Autodesk Inventor part; units mm, degrees
ref_plane "YZ Plane" through (0, 0, 0) normal (1, 0, 0) x (0, 1, 0)
ref_plane "XZ Plane" through (0, 0, 0) normal (0, 1, 0) x (-1, 0, 0)
ref_plane "XY Plane" through (0, 0, 0) normal (0, 0, 1) x (1, 0, 0)
sketch "Sketch1" plane through (0, 0, 0) normal (0, 0, 1) x (1, 0, 0)
  circle A0 centre (190.0545, 3.9636) radius 5.5
  circle A1 centre (-96.9878, 447.3295) radius 5.5
  arc A2 (177.463, -4.1883) -> (202.646, 12.1156) centre (190.0545, 3.9636) ccw
  arc A3 (-84.3963, 455.4815) -> (-109.5793, 439.1776) centre (-96.9878, 447.3295) ccw
  line L0 (-84.3963, 455.4815) -> (202.646, 12.1156)
  line L1 (177.463, -4.1883) -> (-109.5793, 439.1776)
  circle A4 centre (190.0545, 3.9636) radius 5.5
  circle A5 centre (-96.9878, 447.3295) radius 5.5
  point P0 (0, 0)
  dimension "d2" = 30
  dimension "d3" = 30
  dimension "d4" = 11
  dimension "d5" = 11
extrude "Extrusion2" add sketch "Sketch1" along normal blind 6
properties material "Steel, Mild"
Input: part model. Units: mm. Frame: model coordinates. Give positions to 0.01 mm unless a question says otherwise; leave off trailing zeros. Loops run counter-clockwise (first coordinate to the right, second up) from the corner with the lowest first, then second, coordinate; pieces in that order, holes last. Notation, with made-up numbers: M 76,77 L 84,77 A20 ccw 84,102 Z; hole C 89.25,77.25 d4. An arc over 180 degrees is marked long. Use CSV: the item, a comma, the result in double quotes.
(1) Pin query (flat end, axial travel): P1, Ø2, axis at x = 9.5, z = 5.5, coming from the -Y side; P2, Ø1.5, axis at x = 135.5, z = 2, coming from the +Y side; P3, Ø1.5, axis at x = 47, z = 1.5, coming from the -Y side. Return the tip coordinate at first contact, or that it passes through.
Outcome:
P1,"stops at y = 253.7"
P2,"stops at y = 116.99"
P3,"stops at y = 196.17"
(2) Pull-direction query (X, two-part tool) for faces 1 (the face through (57.116, 236.902, 2.958)), 2 (the face through (46, 227, 0)), 3 (the face through (195.3, 2.31, 2.96)); classes: pulls with the +X half, pulls with the -X half, needs draft (parallel to the pull), parting line crosses it, or undercut.
Outcome:
face 1,"pulls with the +X half"
face 2,"needs draft"
face 3,"undercut"
(3) Material intervals for L1, parallel to Y at x = 23, z = 2.55; L2, parallel to Y at x = -64, z = 1.3; L3, parallel to X at y = 316, z = 3.6, sorted ascending. Write a range as [from, to].
Outcome:
L1,"y = [234.4, 289.6]"
L2,"y = [368.78, 423.98]"
L3,"x = [-29.83, 5.91]"
(4) Section C-C, the plane x = 48. Return loops of the section in (y, z), plus the area to 3 significant figures.
Outcome:
outline,"M 195.78,0 L 250.98,0 L 250.98,6 L 195.78,6 Z"
area,"331 mm²"
(5) Section A-A, the plane z = 3.75. Return loops of the section in (x, y), plus the area to 3 significant figures.
Outcome:
outline,"M -109.58,439.18 L 177.46,-4.19 A15 ccw 202.65,12.12 L -84.4,455.48 A15 ccw Z; hole C -96.99,447.33 d11; hole C 190.05,3.96 d11"
area,"16,400 mm²"
(6) Section B-B, the plane y = 31. Return loops of the section in (x, z), plus the area to 3 significant figures.
Outcome:
outline,"M 154.68,0 L 190.42,0 L 190.42,6 L 154.68,6 Z"
area,"214 mm²"
